from build123d import *

# Parameters (mm, degrees)
SKETCH1_W           = 50
SKETCH1_H           = 40
BOSS_EXTRUDE1_DEPTH = 40
CUT_EXTRUDE1_DEPTH  = 30
CUT_EXTRUDE2_DEPTH  = 10
CUT_EXTRUDE3_DEPTH  = 10


with BuildPart() as part:
    # Sketch1 → Boss-Extrude1 (new body)
    with BuildSketch(Plane(origin=(0, 0, 0), x_dir=(1, 0, 0), z_dir=(0, 1, 0))):
        Rectangle(SKETCH1_W, SKETCH1_H)
    extrude(amount=BOSS_EXTRUDE1_DEPTH)

    # Sketch3 → Cut-Extrude1 (cut)
    with BuildSketch(Plane.XY.offset(20)):
        Polygon((-15, 40), (-15, 30), (-5, 30), (-5, 20), (25, 20), (25, 40), align=None)
    extrude(amount=-CUT_EXTRUDE1_DEPTH, mode=Mode.SUBTRACT)

    # Sketch4 → Cut-Extrude2 (cut)
    with BuildSketch(Plane(origin=(0, 20, 0), x_dir=(1, 0, 0), z_dir=(0, 1, 0))):
        Polygon((15, 10), (5, -20), (25, -20), (25, 10), align=None)
    extrude(amount=-CUT_EXTRUDE2_DEPTH, mode=Mode.SUBTRACT)

    # Sketch5 → Cut-Extrude3 (cut)
    with BuildSketch(Plane.XY.offset(-10)):
        Polygon((5, 40), (25, 20), (25, 40), align=None)
    extrude(amount=-CUT_EXTRUDE3_DEPTH, mode=Mode.SUBTRACT)


solid = part.part
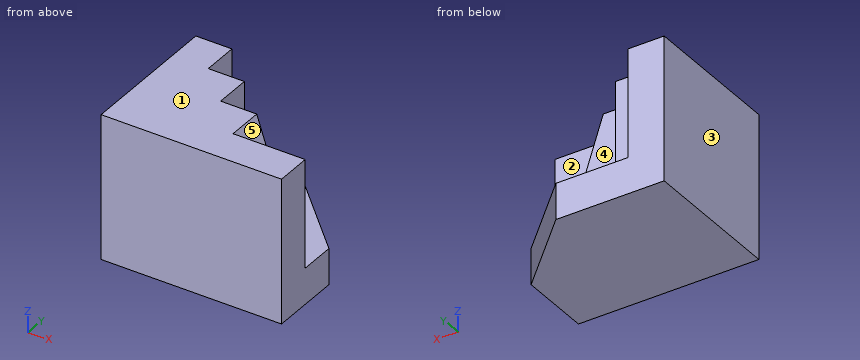
CAD build for the part. Positions are in the model's coordinates, mm. Face numbers are marked on the shaded views. A direction names the side the tool comes from. Give positions to 0.01 mm unless a question says otherwise; leave off trailing zeros. Loops run counter-clockwise (first coordinate to the right, second up) from the corner with the lowest first, then second, coordinate; pieces in that order, holes last. Notation, with made-up numbers: M 9,-9.5 L 15,-9.5 A29 cw 15,10.5 Z; hole C 72,20.25 d1. An arc over 180 degrees is marked long. One line per question, with ' | ' between items. Start each with the question number.
1. Saw through at D-D on z = -7. Give the cut face in (x, y), plus the area to 3 significant figures.
2. Saw through at B-B on z = -1. Give the cut face in (x, y).
3. Probe L1, parallel to X at y = 34, z = 13; L2, parallel to Y at x = -6, z = 6.5; L3, parallel to Y at x = -3, z = 6.5. List the from-to ranges inside material, lowest first. Write a range as from..to.
4. Flat gauge pins, fed straight in: pin 1 (10 mm diameter, centred on x = 10.5, z = 0, fed in from +Y); pin 2 (11 mm diameter, centred on y = 27, z = 12, fed in from +X); pin 3 (8 mm diameter, centred on x = -10.5, z = 6.5, fed in from +Y). Where does each tip first touch, or does it go through?
5. 3-axis set-ups, long thin cutter, end or side, ignore diameter. For the marked faces 1 and 2: which of +Z, -Z, +X, -X, +Y, -Y reach the whole face in a straight line?
6. Two-plate mould, pull along X, no slides. Class the marked faces 3, 4 and 5: pulls with the +X half, pulls with the -X half, needs draft (parallel to the pull), parting line crosses it, or undercut.
7. Saw through at A-A on x = 6.5. Give the cut face in (y, z).
8. Saw through at C-C on y = 21.5. Give the cut face in (x, z).
Result sheet:
1) outline: M -25,0 L 25,0 L 25,10 L 14,10 L 14,20 L -5,20 L -5,30 L -15,30 L -15,40 L -25,40 Z | area: 1,190 mm^2
2) outline: M -25,0 L 25,0 L 25,10 L 12,10 L 12,20 L -5,20 L -5,30 L -15,30 L -15,40 L -25,40 Z
3) L1: x = -25..-15 | L2: y = 0..30 | L3: y = 0..20
4) pin 1: stops at y = 20 | pin 2: stops at x = -5 | pin 3: stops at y = 30
5) face 1: +Z, +X, -X, +Y, -Y | face 2: +Z, +X, +Y
6) face 3: pulls with the -X half | face 4: needs draft | face 5: pulls with the +X half
7) outline: M 0,-20 L 38.5,-20 L 38.5,-10 L 20,-10 L 20,15.5 L 10,15.5 L 10,20 L 0,20 Z
8) outline: M -25,-20 L 23.5,-20 L 23.5,-10 L -5,-10 L -5,20 L -25,20 Z
